Could you check a few things on this model? Use its own coordinates, in mm. A direction names the side the tool comes from. Give positions to 0.01 mm unless a question says otherwise; leave off trailing zeros. Loops run counter-clockwise (first coordinate to the right, second up) from the corner with the lowest first, then second, coordinate; pieces in that order, holes last. Notation, with made-up numbers: (9.5, -34.5) -> (51.5, -34.5) arc R24 cw to (51.5, 1.5) -> close; hole circle Ø3 at (-8, -18.75). An arc over 180 degrees is marked (long way). Write each question's results on one line, items separated by ' | '. Start each with the question number.
Q1. If I drill on line 1 along X through (y, z) = (4.85, -4); line 2 along X through (y, z) = (3.6, -50); line 3 along Z through (x, y) = (-55.5, 3.4), over which ranges is the centre line in solid material (lowest first)?
Q2. If we section it at A-A, the plane x = -56.5: List the corners of the cut face in (y, z) for me.
Q3. If we section it at B-B, the plane z = -3: List the corners of the cut face in (x, y) for me.
Q4. If we section it at C-C, the plane z = 30: List the corners of the cut face in (x, y) for me, plus the area to 3 significant figures.
Q5. We'd pull the mould along Z, two halves only. Please class faces 1 (the face through (-96, 3, -5)), 2 (the face through (104, 2, 1)), 3 (the face through (-1, 2, -90)): released by +Z, released by -Z, zero draft, split by the parting line, or undercut.
Q6. Will this pin go through, and if not, where does the flat tip stop? P1, Ø5, axis at x = 0, z = 65, coming from the -Y side.
Q7. Which directions (+Z, -Z, +X, -X, +Y, -Y) give clear straight access to the entire face, cutting with the end or side of a thin tool? Please do faces 4 (the face through (-8, 3, 20)), 5 (the face through (-1, 2, 90)).
Q8. If we section it at D-D, the plane y = 2.7: Give the number of separate pieces and of enclosed holes in the cut face, plus the area to 3 significant figures.
from build123d import *

# Parameters (mm, degrees)
D_KESIM_W                   = 208
D_KESIM_H                   = 180
ANA_PLAKA_DEPTH             = 5
BASEBOARD_PI_R              = 1.6
BASE_PI_DEPTH               = 6
KASA_BA_LANT_LAR_DEPTH      = 6
SKETCH3_R                   = 3
LIPO_YUVAS_DEPTH            = 6
SKETCH1_R                   = 1.6
MAINBOARD_DEPTH             = 6
SKETCH5_R                   = 2.1
VIDA_DELIKLERI_DEPTH        = 6
KABLO_AKTAR_M_BO_LU_U_DEPTH = 6
SHARP_SENSOR_DEPTH          = 6
SKETCH11_R                  = 3.05
STOP_BUTON_DEPTH            = 6
SKETCH10_R                  = 1.6
MOTOR_DRIVER_DEPTH          = 6


with BuildPart() as part:
    # Dış Kesim → Ana Plaka (new body)
    with BuildSketch(Plane(origin=(0, 0, 0), x_dir=(1, 0, 0), z_dir=(0, 1, 0))):
        Rectangle(D_KESIM_W, D_KESIM_H)
    extrude(amount=ANA_PLAKA_DEPTH)

    # BaseBoard + Pi → Base - Pi (cut, through all)
    with BuildSketch(Plane(origin=(0, 0, 0), x_dir=(1, 0, 0), z_dir=(0, 1, 0))):
        with Locations((-30, 50)):
            Circle(BASEBOARD_PI_R)
        with Locations((-79, 50)):
            Circle(BASEBOARD_PI_R)
        with Locations((-79, -8)):
            Circle(BASEBOARD_PI_R)
    extrude(amount=BASE_PI_DEPTH, mode=Mode.SUBTRACT)

    # Sketch2 → Kasa Bağlantıları (cut, through all)
    with BuildSketch(Plane(origin=(0, 5, 0), x_dir=(1, 0, 0), z_dir=(0, 1, 0))):
        with BuildLine():
            Line((-82.15, 35.5), (-82.15, 40.5))
            ThreePointArc((-82.15, 40.5), (-80, 42.65), (-77.85, 40.5))
            Line((-77.85, 40.5), (-77.85, 35.5))
            ThreePointArc((-77.85, 35.5), (-80, 33.35), (-82.15, 35.5))
        make_face()
        with BuildLine():
            Line((-82.35, -42.85), (-82.35, -39.15))
            ThreePointArc((-82.35, -39.15), (-80.5, -37.3), (-78.65, -39.15))
            Line((-78.65, -39.15), (-78.65, -42.85))
            ThreePointArc((-78.65, -42.85), (-80.5, -44.7), (-82.35, -42.85))
        make_face()
        with BuildLine():
            Line((79.65, -41.85), (79.65, -38.15))
            ThreePointArc((79.65, -38.15), (81.5, -36.3), (83.35, -38.15))
            Line((83.35, -38.15), (83.35, -41.85))
            ThreePointArc((83.35, -41.85), (81.5, -43.7), (79.65, -41.85))
        make_face()
        with BuildLine():
            Line((79.15, 36.15), (79.15, 39.85))
            ThreePointArc((79.15, 39.85), (81, 41.7), (82.85, 39.85))
            Line((82.85, 39.85), (82.85, 36.15))
            ThreePointArc((82.85, 36.15), (81, 34.3), (79.15, 36.15))
        make_face()
    extrude(amount=-KASA_BA_LANT_LAR_DEPTH, mode=Mode.SUBTRACT)

    # Sketch3 → LiPo Yuvası (cut, through all)
    with BuildSketch(Plane(origin=(0, 5, 0), x_dir=(1, 0, 0), z_dir=(0, 1, 0))):
        with Locations((14, -30)):
            Circle(SKETCH3_R)
        with BuildLine():
            Line((-59, 25), (-68, 25))
            ThreePointArc((-68, 25), (-70.121320344, 24.121320344), (-71, 22))
            Line((-71, 22), (-71, -17))
            ThreePointArc((-71, -17), (-70.121320344, -19.121320344), (-68, -20))
            Line((-68, -20), (53, -20))
            ThreePointArc((53, -20), (55.121320344, -20.878679656), (56, -23))
            Line((56, -23), (56, -37))
            ThreePointArc((56, -37), (56.878679656, -39.121320344), (59, -40))
            Line((59, -40), (68, -40))
            ThreePointArc((68, -40), (70.121320344, -39.121320344), (71, -37))
            Line((71, -37), (71, -15))
            Line((71, -15), (71, 22))
            ThreePointArc((71, 22), (70.121320344, 24.121320344), (68, 25))
            Line((68, 25), (-59, 25))
        make_face()
        with BuildLine():
            Line((-68, -24), (-49, -24))
            ThreePointArc((-49, -24), (-46.878679656, -24.878679656), (-46, -27))
            Line((-46, -27), (-46, -36))
            ThreePointArc((-46, -36), (-46.878679656, -38.121320344), (-49, -39))
            Line((-49, -39), (-68, -39))
            ThreePointArc((-68, -39), (-70.121320344, -38.121320344), (-71, -36))
            Line((-71, -36), (-71, -27))
            ThreePointArc((-71, -27), (-70.121320344, -24.878679656), (-68, -24))
        make_face()
    extrude(amount=-LIPO_YUVAS_DEPTH, mode=Mode.SUBTRACT)

    # Sketch1 → MainBoard (cut, through all)
    with BuildSketch(Plane(origin=(0, 5, 0), x_dir=(1, 0, 0), z_dir=(0, 1, 0))):
        with Locations((-12, 29.5)):
            Circle(SKETCH1_R)
        with Locations((75, 29.5)):
            Circle(SKETCH1_R)
        with Locations((75, -25.5)):
            Circle(SKETCH1_R)
        with Locations((-12, -25.5)):
            Circle(SKETCH1_R)
    extrude(amount=-MAINBOARD_DEPTH, mode=Mode.SUBTRACT)

    # Sketch5 → Vida Delikleri (cut, through all)
    with BuildSketch(Plane(origin=(0, 5, 0), x_dir=(1, 0, 0), z_dir=(0, 1, 0))):
        with Locations((-74, 70)):
            Circle(SKETCH5_R)
        with Locations((74, 70)):
            Circle(SKETCH5_R)
        with Locations((74, -70)):
            Circle(SKETCH5_R)
        with Locations((-74, -70)):
            Circle(SKETCH5_R)
    extrude(amount=-VIDA_DELIKLERI_DEPTH, mode=Mode.SUBTRACT)

    # Sketch8 → Kablo Aktarım Boşluğu (cut, through all)
    with BuildSketch(Plane(origin=(0, 5, 0), x_dir=(1, 0, 0), z_dir=(0, 1, 0))):
        with BuildLine():
            Line((68, 41), (39, 41))
            ThreePointArc((39, 41), (36.878679656, 40.121320344), (36, 38))
            Line((36, 38), (36, 31))
            ThreePointArc((36, 31), (36.878679656, 28.878679656), (39, 28))
            Line((39, 28), (68, 28))
            ThreePointArc((68, 28), (70.121320344, 28.878679656), (71, 31))
            Line((71, 31), (71, 38))
            ThreePointArc((71, 38), (70.121320344, 40.121320344), (68, 41))
        make_face()
    extrude(amount=-KABLO_AKTAR_M_BO_LU_U_DEPTH, mode=Mode.SUBTRACT)

    # Sketch9 → Sharp Sensor (cut, through all)
    with BuildSketch(Plane(origin=(0, 5, 0), x_dir=(1, 0, 0), z_dir=(0, 1, 0))):
        with BuildLine():
            Line((-94, 12.5), (-86, 12.5))
            ThreePointArc((-86, 12.5), (-84.585786438, 11.914213562), (-84, 10.5))
            Line((-84, 10.5), (-84, -0.5))
            ThreePointArc((-84, -0.5), (-84.585786438, -1.914213562), (-86, -2.5))
            Line((-86, -2.5), (-94, -2.5))
            ThreePointArc((-94, -2.5), (-95.414213562, -1.914213562), (-96, -0.5))
            Line((-96, -0.5), (-96, 10.5))
            ThreePointArc((-96, 10.5), (-95.414213562, 11.914213562), (-94, 12.5))
        make_face()
        with BuildLine():
            Line((95, 7.5), (87, 7.5))
            ThreePointArc((87, 7.5), (85.585786438, 6.914213562), (85, 5.5))
            Line((85, 5.5), (85, -5.5))
            ThreePointArc((85, -5.5), (85.585786438, -6.914213562), (87, -7.5))
            Line((87, -7.5), (95, -7.5))
            ThreePointArc((95, -7.5), (96.414213562, -6.914213562), (97, -5.5))
            Line((97, -5.5), (97, 5.5))
            ThreePointArc((97, 5.5), (96.414213562, 6.914213562), (95, 7.5))
        make_face()
    extrude(amount=-SHARP_SENSOR_DEPTH, mode=Mode.SUBTRACT)

    # Sketch11 → Stop Buton (cut, through all)
    with BuildSketch(Plane(origin=(0, 5, 0), x_dir=(1, 0, 0), z_dir=(0, 1, 0))):
        with Locations((0, -65)):
            Circle(SKETCH11_R)
    extrude(amount=-STOP_BUTON_DEPTH, mode=Mode.SUBTRACT)

    # Sketch10 → Motor Driver (cut, through all)
    with BuildSketch(Plane(origin=(0, 5, 0), x_dir=(1, 0, 0), z_dir=(0, 1, 0))):
        with Locations((-11.5, 40)):
            Circle(SKETCH10_R)
        with Locations((22.5, 40)):
            Circle(SKETCH10_R)
        with Locations((-11.5, 79)):
            Circle(SKETCH10_R)
        with Locations((22.5, 79)):
            Circle(SKETCH10_R)
    extrude(amount=-MOTOR_DRIVER_DEPTH, mode=Mode.SUBTRACT)


solid = part.part
Final values:
1) line 1: x = -104 to -96, -84 to -71, 71 to 85, 97 to 104 | line 2: x = -104 to -80.6, -77.4 to -31.6, -28.4 to 104 | line 3: z = -90 to -25, 20 to 24, 39 to 90
2) outline: (0, -90) -> (5, -90) -> (5, -25) -> (0, -25) -> close; (0, 20) -> (5, 20) -> (5, 24) -> (0, 24) -> close; (0, 39) -> (5, 39) -> (5, 90) -> (0, 90) -> close
3) outline: (-104, 0) -> (-96, 0) -> (-96, 5) -> (-104, 5) -> close; (-84, 0) -> (-71, 0) -> (-71, 5) -> (-84, 5) -> close; (71, 0) -> (85, 0) -> (85, 5) -> (71, 5) -> close; (97, 0) -> (104, 0) -> (104, 5) -> (97, 5) -> close
4) outline: (-104, 0) -> (-71, 0) -> (-71, 5) -> (-104, 5) -> close; (-46, 0) -> (11, 0) -> (11, 5) -> (-46, 5) -> close; (17, 0) -> (56, 0) -> (56, 5) -> (17, 5) -> close; (71, 0) -> (104, 0) -> (104, 5) -> (71, 5) -> close | area: 810 mm²
5) face 1: undercut | face 2: zero draft | face 3: released by -Z
6) P1: passes through
7) face 4: +Y, -Y | face 5: +Z, +X, -X, +Y, -Y
8) separate pieces: 1 | enclosed holes: 26 | area: 29,300 mm²
